Geometry: final body of the model. Coordinates: model frame, mm. Face numbers are marked on the shaded views. A direction names the side the tool comes from. Give positions to 0.01 mm unless a question says otherwise; leave off trailing zeros. Write each loop counter-clockwise with the first axis right and the second up, starting at its lowest first coordinate (ties: lowest second). Pieces come first, ordered by that corner, then holes.
Q1. Section D-D (y = 16.5). Return the cut outline in (x, z), plus the area to 3 significant figures.
Q2. Line query: line 1 (Y direction, x = 18, z = 4.2); line 2 (X direction, y = 14.5, z = 0.7); line 3 (Y direction, x = 37, z = 2.1). Output: solid intervals per line, ascending.
Q3. Reachability of the marked faces 5, 6 and 7 from +Z, -Z, +X, -X, +Y, -Y: full face, straight path, thin tool, end or side. Return the list, or none.
Q4. Section B-B (y = 5). Return the cut outline in (x, z), plus the area to 3 significant figures.
Q5. Mould query, pull axis Y, two halves, no side actions, for the marked faces 1, 2, 3 and 4. Classes: +Y half, -Y half, draft (parallel to the pull), parting line (faces both ways), or undercut.
Q6. Pin query (flat end, axial travel): pin 1 Ø2 at (x, z) = (4, 3) entering from +Y; pin 2 Ø0.9 at (x, z) = (2, 3) entering from -Y; pin 3 Ø2.5 at (x, z) = (32, 3) entering from +Y. Return the tip coordinate at first contact, or that it passes through.
Q7. Section A-A (x = 17.9). Return the cut outline in (y, z), plus the area to 3 significant figures.
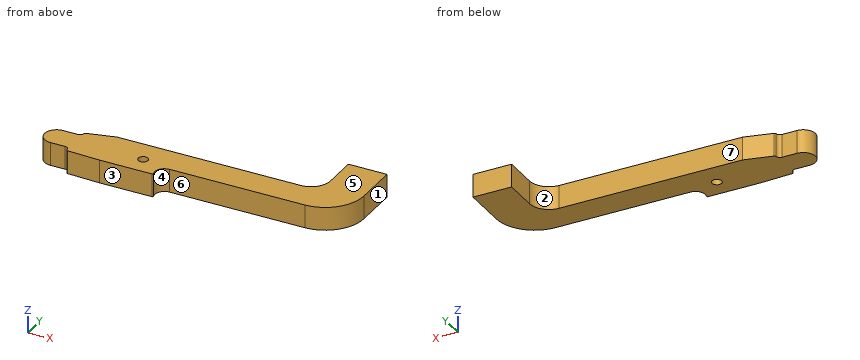
from build123d import *

# Parameters (mm, degrees)
F0_R     = 1
F1_DEPTH = 4.8


with BuildPart() as f1:
    # F0 (on Top) → F1 (new body)
    with BuildSketch(Plane.XY):
        with BuildLine():
            ThreePointArc((51.9, 4), (57.556854, 6.343146), (59.9, 12))
            Line((59.9, 12), (59.9, 21))
            Line((59.9, 21), (51.9, 21))
            Line((51.9, 21), (51.9, 14))
            ThreePointArc((51.9, 14), (50.728427, 11.171573), (47.9, 10))
            Line((47.9, 10), (9.9, 10))
            Line((9.9, 10), (4.202064, 8.561127))
            ThreePointArc((4.202064, 8.561127), (3.984426, 8.419092), (3.9, 8.173302))
            Line((3.9, 8.173302), (3.9, 8.3))
            ThreePointArc((3.9, 8.3), (3.665685, 7.734315), (3.1, 7.5))
            Line((3.1, 7.5), (0, 7.5))
            ThreePointArc((0, 7.5), (-2.5, 5), (0, 2.5))
            Line((0, 2.5), (3.1, 2.5))
            ThreePointArc((3.1, 2.5), (3.665685, 2.265685), (3.9, 1.7))
            Line((3.9, 1.7), (3.9, 1.682928))
            ThreePointArc((3.9, 1.682928), (3.987383, 1.433388), (4.211352, 1.292875))
            Line((4.211352, 1.292875), (11, 1))
            Line((11, 1), (21.85061, 1))
            ThreePointArc((21.85061, 1), (22.015754, 1.087185), (22.036918, 1.272727))
            ThreePointArc((22.036918, 1.272727), (22.248554, 3.128152), (23.9, 4))
            Line((23.9, 4), (51.9, 4))
        make_face()
        with Locations((17.9, 5)):
            Circle(F0_R, mode=Mode.SUBTRACT)
    extrude(amount=F1_DEPTH)


solid = f1.part
Computed:
1. outline: (51.9, 0) - (59.9, 0) - (59.9, 4.8) - (51.9, 4.8) - close
1. area: 38.4 mm2
2. line 1: y = 1 to 4.01, 5.99 to 10
2. line 2: x = 51.9 to 59.9
2. line 3: y = 4 to 10
3. face 5: +Z, +X, -X, +Y, -Y
3. face 6: +Z, -Z, +X, -Y
3. face 7: +Z, -Z, -X, +Y
4. outline: (-2.5, 0) - (16.9, 0) - (16.9, 4.8) - (-2.5, 4.8) - close; (18.9, 0) - (55.77, 0) - (55.77, 4.8) - (18.9, 4.8) - close
4. area: 270 mm2
5. face 1: draft
5. face 2: +Y half
5. face 3: -Y half
5. face 4: undercut
6. pin 1: stops at y = 8.76
6. pin 2: stops at y = 2.5
6. pin 3: stops at y = 10
7. outline: (1, 0) - (4, 0) - (4, 4.8) - (1, 4.8) - close; (6, 0) - (10, 0) - (10, 4.8) - (6, 4.8) - close
7. area: 33.6 mm2
